For this review, use the dimensioned drawing (mm, ordinates from the lowest corner) and the shaded views. A direction names the side the tool comes from. Round coordinates to 2 decimals unless told otherwise and drop trailing zeros. Order: outer loops, then holes, each group sorted by start corner. A loop starts at its lowest first (then second) coordinate and runs counter-clockwise, first axis right, second up. Notation, with made-up numbers: (10, 69.5) - (58, 69.5) arc R21 cw to (58, 76.5) - close; hole circle Ø4 at (83, -22.5). An arc over 180 degrees is marked (long way). Write each question's results on one line, items separated by ' | '. Start each with the question number.
(1) Take a section at A-A, the plane x = 30. Give the boundary of the cut face in (y, z), plus the area to 3 significant figures.
(2) Insertion check: pin 1 Ø12 at (x, z) = (50.5, 43.5) entering from -Y; pin 2 Ø4 at (y, z) = (42.5, 17) entering from -X; pin 3 Ø20 at (x, z) = (18.5, 79.5) entering from +Y; pin 4 Ø12.5 at (x, z) = (15.5, 53) entering from -Y. Each pin has a flat end and moves straight along its axis. Give the tip position at first contact, or say it passes through.
(3) Take a section at B-B, the plane y = 15. Give the boundary of the cut face in (x, z), plus the area to 3 significant figures.
(4) For the marked faces 1, 2, 3, 4 and 5, list the 3-axis set-ups (+Z, -Z, +X, -X, +Y, -Y) from which the entire face can be reached by the end or side of a thin tool; tool diameter is ignored.
(5) For L1, parallel to Y at x = 30, z = 16; L2, parallel to X at y = 60, z = 45; L3, parallel to Y at x = 10.5, z = 40.5, list the stretches that pass through material, from the lowest coordinate up. Write a range as from..to.
(6) Take a section at D-D, the plane z = 16.5. Give the boundary of the cut face in (x, y), plus the area to 3 significant figures.
(7) Take a section at C-C, the plane x = 8.5. Give the boundary of the cut face in (y, z).
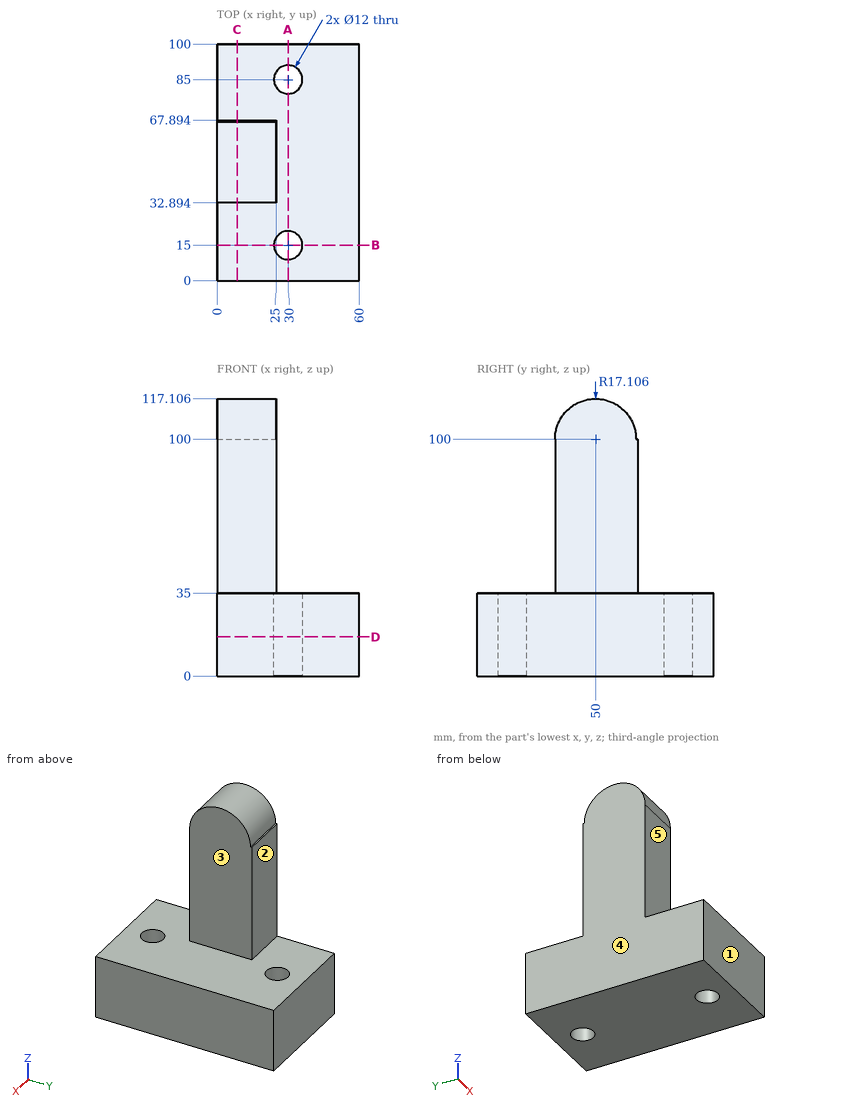
Results below:
1) outline: (0, 0) - (9, 0) - (9, 35) - (0, 35) - close; (21, 0) - (79, 0) - (79, 35) - (21, 35) - close; (91, 0) - (100, 0) - (100, 35) - (91, 35) - close | area: 2,660 mm^2
2) pin 1: passes through | pin 2: stops at x = 0 | pin 3: stops at y = 67.89 | pin 4: stops at y = 32.89
3) outline: (0, 0) - (24, 0) - (24, 35) - (0, 35) - close; (36, 0) - (60, 0) - (60, 35) - (36, 35) - close | area: 1,680 mm^2
4) face 1: +Z, -Z, +X, -X, -Y | face 2: +Z, +X, -X, +Y | face 3: +Z, +X, +Y, -Y | face 4: +Z, -Z, -X, +Y, -Y | face 5: +Z, +X, -X, -Y
5) L1: y = 0..9, 21..79, 91..100 | L2: x = 0..25 | L3: y = 32.89..67.89
6) outline: (0, 0) - (60, 0) - (60, 100) - (0, 100) - close; hole circle Ø12 at (30, 15); hole circle Ø12 at (30, 85) | area: 5,770 mm^2
7) outline: (0, 0) - (100, 0) - (100, 35) - (67.89, 35) - (67.89, 100) - (67.11, 100) arc R17.11 ccw to (32.89, 100) - (32.89, 35) - (0, 35) - close
